```python
from build123d import *

# Parameters (mm, degrees)
F0_W     = 120
F0_H     = 150
F1_DEPTH = 3
F3_DEPTH = 750
F5_DEPTH = 2
F7_DEPTH = 2


with BuildPart() as f1:
    # F0 (on Front) → F1 (new body)
    with BuildSketch(Plane.XZ):
        Rectangle(F0_W, F0_H)
    extrude(amount=-F1_DEPTH)

    # F2 (on face) → F3 (join)
    with BuildSketch(Plane.XZ):
        Polygon((-23, 19.26168), (-15, 19.26168), (-15, 21.26168), (-25, 21.26168), (-25, -25), (25, -25), (25, 21.26168), (15, 21.26168), (15, 19.26168), (23, 19.26168), (23, -23), (-23, -23), align=None)
    extrude(amount=F3_DEPTH)

    # F4 (on face) → F5 (join)
    with BuildSketch(Plane.YZ.offset(25)):
        Polygon((-50, -25), (0, -75), (0, 75), (-50, 21.26168), align=None)
    extrude(amount=F5_DEPTH)

    # F6 (on face) → F7 (join)
    with BuildSketch(Plane(origin=(-25, 0, 0), x_dir=(0, -1, 0), z_dir=(-1, 0, 0))):
        Polygon((0, 75), (0, -75), (50, -25), (50, 21.26168), align=None)
    extrude(amount=F7_DEPTH)


solid = f1.part
```
Geometry check sheet. Reference: the model listing, model coordinates, mm. A direction names the side the tool comes from. Round coordinates to 2 decimals unless told otherwise and drop trailing zeros. Loops run counter-clockwise (first coordinate to the right, second up) from the corner with the lowest first, then second, coordinate; pieces in that order, holes last. Notation, with made-up numbers: (-25, 9) - (-4, 9) arc R15 cw to (-4, 17) - close; hole circle Ø11 at (83.5, 38.25). An arc over 180 degrees is marked (long way). Use a Markdown table: item, result.
Q1. Material ranges on line 1 (X direction, y = -513, z = -5); line 2 (Z direction, x = 20.5, y = -568); line 3 (Y direction, x = 23, z = -25.5), recorded low to high.
Solutions:
| item | result |
|---|---|
| line 1 | x = -25 to -23, 23 to 25 |
| line 2 | z = -25 to -23, 19.26 to 21.26 |
| line 3 | y = 0 to 3 |
Q2. Cross-section at A-A on y = -468. Record the cut outline in (x, z), plus the area to 3 significant figures.
Solutions:
| item | result |
|---|---|
| outline | (-25, -25) - (25, -25) - (25, 21.26) - (15, 21.26) - (15, 19.26) - (23, 19.26) - (23, -23) - (-23, -23) - (-23, 19.26) - (-15, 19.26) - (-15, 21.26) - (-25, 21.26) - close |
| area | 309 mm2 |
Q3. Access from +Z, -Z, +X, -X, +Y, -Y to the whole of each face (thin tool, end or side, straight path). Record for faces 1 (the flat face through (-44, 0, 1)), 2 (the flat face through (43, 0, 1)), 3 (the flat face through (0, -370, -23)), 4 (the flat face through (-25, -19, -44)).
Solutions:
| item | result |
|---|---|
| face 1 | +Z, -Z, -X, -Y |
| face 2 | +Z, -Z, +X, -Y |
| face 3 | -Y |
| face 4 | -Z, -Y |
Q4. Draft check along X on faces 5 (the flat face through (-25, -395, -2)), 6 (the flat face through (-25, -14, 37)), 7 (the flat face through (-1, 3, 1)). Enter one of: released by +X, released by -X, zero draft, split by the parting line, or undercut.
Solutions:
| item | result |
|---|---|
| face 5 | released by -X |
| face 6 | undercut |
| face 7 | zero draft |
Q5. Go/stop test with flat-tipped pins: P1, Ø8, axis at x = 19, y = -620, coming from the -Z side; P2, Ø10, axis at x = 50.5, z = -3.5, coming from the -Y side; P3, Ø10, axis at x = 24.5, z = 38, coming from the -Y side. Record where each tip stops, or that it passes through.
Solutions:
| item | result |
|---|---|
| P1 | stops at z = -25 |
| P2 | stops at y = 0 |
| P3 | stops at y = -39.05 |
Q6. Cross-section at D-D on z = -6.5. Record the cut outline in (x, y), plus the area to 3 significant figures.
Solutions:
| item | result |
|---|---|
| outline | (-60, 0) - (-27, 0) - (-27, -50) - (-25, -50) - (-25, -750) - (-23, -750) - (-23, 0) - (23, 0) - (23, -750) - (25, -750) - (25, -50) - (27, -50) - (27, 0) - (60, 0) - (60, 3) - (-60, 3) - close |
| area | 3,560 mm2 |
Q7. Cross-section at B-B on x = 6. Record the cut outline in (y, z).
Solutions:
| item | result |
|---|---|
| outline | (-750, -25) - (0, -25) - (0, -75) - (3, -75) - (3, 75) - (0, 75) - (0, -23) - (-750, -23) - close |
Q8. Cross-section at C-C on z = -63. Record the cut outline in (x, y), plus the area to 3 significant figures.
Solutions:
| item | result |
|---|---|
| outline | (-60, 0) - (-27, 0) - (-27, -12) - (-25, -12) - (-25, 0) - (25, 0) - (25, -12) - (27, -12) - (27, 0) - (60, 0) - (60, 3) - (-60, 3) - close |
| area | 408 mm2 |
